The listing builds one solid part. Answer for the finished solid, in the listing's coordinates (mm). A direction names the side the tool comes from. Give positions to 0.01 mm unless a question says otherwise; leave off trailing zeros. Loops run counter-clockwise (first coordinate to the right, second up) from the corner with the lowest first, then second, coordinate; pieces in that order, holes last. Notation, with made-up numbers: (14, -15.75) -> (34, -15.75) arc R22 ccw to (34, 11.25) -> close; hole circle Ø9 at (40, -1.75). An arc over 180 degrees is marked (long way). One line per question, with ' | ' between items. Start each with the question number.
from build123d import *

# Parameters (mm, degrees)
F1_DEPTH = 50
F2_R     = 35
F3_DEPTH = 200


with BuildPart() as f1:
    # F0 (on Top) → F1 (new body, symmetric)
    with BuildSketch(Plane.XY):
        with BuildLine():
            Line((5, 39.68627), (-5, 39.68627))
            ThreePointArc((-5, 39.68627), (-28.427655, 28.140156), (-39.735042, 4.596351))
            ThreePointArc((-39.735042, 4.596351), (-39.999989, -0.030145), (-39.728069, -4.656237))
            ThreePointArc((-39.728069, -4.656237), (-28.434455, -28.133286), (-5.078989, -39.676238))
            ThreePointArc((-5.078989, -39.676238), (-0.14475, -39.999738), (4.791701, -39.711958))
            ThreePointArc((4.791701, -39.711958), (27.854373, -28.707732), (39.54933, -5.987525))
            ThreePointArc((39.54933, -5.987525), (39.997358, -0.45972), (39.676503, 5.076922))
            ThreePointArc((39.676503, 5.076922), (28.256844, 28.311672), (5, 39.68627))
        make_face()
        with BuildLine():
            ThreePointArc((-39.735042, 4.596351), (-28.427655, 28.140156), (-5, 39.68627))
            Line((-5, 39.68627), (-5, 49.749372))
            ThreePointArc((-5, 49.749372), (-35.355339, 35.355339), (-49.749372, 5))
            Line((-49.749372, 5), (-39.735042, 4.596351))
        make_face()
        with BuildLine():
            Line((5, 49.749372), (5, 39.68627))
            ThreePointArc((5, 39.68627), (28.256844, 28.311672), (39.676503, 5.076922))
            Line((39.676503, 5.076922), (49.741581, 5.076922))
            ThreePointArc((49.741581, 5.076922), (35.327993, 35.382664), (5, 49.749372))
        make_face()
        with BuildLine():
            ThreePointArc((-5.078989, -39.676238), (-28.434455, -28.133286), (-39.728069, -4.656237))
            Line((-39.728069, -4.656237), (-49.782722, -4.656237))
            ThreePointArc((-49.782722, -4.656237), (-35.477237, -35.233019), (-5, -49.749372))
            Line((-5, -49.749372), (-5.078989, -39.676238))
        make_face()
        with BuildLine():
            Line((49.640201, -5.987525), (39.54933, -5.987525))
            ThreePointArc((39.54933, -5.987525), (27.854373, -28.707732), (4.791701, -39.711958))
            Line((4.791701, -39.711958), (5, -49.749372))
            ThreePointArc((5, -49.749372), (35.002324, -35.704864), (49.640201, -5.987525))
        make_face()
    extrude(amount=F1_DEPTH, both=True)

    # F2 (on face) → F3 (cut)
    with BuildSketch(Plane.XY.offset(50)):
        Circle(F2_R)
    extrude(amount=-F3_DEPTH, mode=Mode.SUBTRACT)


solid = f1.part
1. Straight lines are drawn through the part: L1, parallel to Y at x = 0, z = -19; L2, parallel to X at y = 12, z = -10.5; L3, parallel to Y at x = -30, z = 37. For each, find the intervals that lie inside material, in ascending order.
2. The part is cut by section B-B (z = 15). Write down the section's boundary in (x, y).
3. Each of these flat-tipped pins is pushed along its axis until it touches: pin 1 Ø3 at (y, z) = (45, 10) entering from -X; pin 2 Ø3 at (x, z) = (-1.5, 3) entering from +Y; pin 3 Ø8 at (x, z) = (-46, -24.5) entering from +Y. Where does it stop, or does it pass through?
4. Determine the mould class of faces 6 (the flat face through (-44.8, 4.8, 0.7)), 7 (the cylindrical face through (-28, -21, 1)), 8 (the cylindrical face through (35.67, 35.04, 0.7)) for opening direction X: released by +X, released by -X, zero draft, split by the parting line, or undercut.
5. The part is cut by section C-C (x = 0). Write down the section's boundary in (y, z).
6. For faces 1 (the flat face through (-12, 34, -50)), 2 (the cylindrical face through (-35.815, -34.889, 0.7)), 3 (the flat face through (45, 5.077, 1)), 4 (the flat face through (-5, 45, 1)), 5 (the flat face through (-45, -4.656, 1)), determine the directions among +Z, -Z, +X, -X, +Y, -Y from which every point of the face is accessible in a straight line to the end or side of a thin tool.
7. The part is cut by section D-D (x = 37). Write down the section's boundary in (y, z), plus the area to 3 significant figures.
8. The part is cut by section A-A (y = 0). Write down the section's boundary in (x, z), plus the area to 3 significant figures.
Check sheet entries:
1) L1: y = -40 to -35, 35 to 39.69 | L2: x = -48.54 to -32.88, 32.88 to 48.54 | L3: y = -40 to -18.03, 18.03 to 40
2) outline: (-49.78, -4.66) arc R50 ccw to (-5, -49.75) -> (-5.08, -39.68) arc R40 ccw to (4.79, -39.71) -> (5, -49.75) arc R50 ccw to (49.64, -5.99) -> (39.55, -5.99) arc R40 ccw to (39.68, 5.08) -> (49.74, 5.08) arc R50 ccw to (5, 49.75) -> (5, 39.69) -> (-5, 39.69) -> (-5, 49.75) arc R50 ccw to (-49.75, 5) -> (-39.74, 4.6) arc R40 ccw to (-39.73, -4.66) -> close; hole circle Ø70 at (0, 0)
3) pin 1: stops at x = -24.65 | pin 2: stops at y = 39.69 | pin 3: stops at y = 27.13
4) face 6: released by -X | face 7: undercut | face 8: released by +X
5) outline: (-40, -50) -> (-35, -50) -> (-35, 50) -> (-40, 50) -> close; (35, -50) -> (39.69, -50) -> (39.69, 50) -> (35, 50) -> close
6) face 1: -Z, +X, -X, +Y, -Y | face 2: +Z, -Z, -X, -Y | face 3: +Z, -Z, +X | face 4: +Z, -Z, +Y | face 5: +Z, -Z, -X
7) outline: (-33.63, -50) -> (33.63, -50) -> (33.63, 50) -> (-33.63, 50) -> close | area: 6,730 mm^2
8) outline: (-40, -50) -> (-35, -50) -> (-35, 50) -> (-40, 50) -> close; (35, -50) -> (40, -50) -> (40, 50) -> (35, 50) -> close | area: 1,000 mm^2
